Read the model definition and answer for the solid it produces. Units are mm, in the model's axes. Face numbers are marked on the shaded views. A direction names the side the tool comes from. Coordinates: 2 decimals unless noted, no trailing zeros. Write each loop counter-clockwise with the first axis right and the second up, starting at its lowest first coordinate (ties: lowest second). Pieces come first, ordered by that corner, then holes. Notation, with made-up numbers: (20.25, -34) -> (77.25, -34) arc R13 ccw to (77.25, -28) -> close; hole circle Ø4 at (-10.75, 88). An arc over 180 degrees is marked (long way). Answer as a JSON object with one key per item and string values. Group by question number.
(1) Which of the six approach directions +Z, -Z, +X, -X, +Y, -Y give full straight-line access (tool end or side, diameter ignored) to the marked faces 1 and 2?
(2) Find section B-B (x = 23.5). Give the vertices of the cut face in (y, z), then the cut area to 3 significant figures.
(3) Find section C-C (z = 12). Give the vertices of the cut face in (x, y).
(4) For a pull along X with two mould halves and no side action, classify the marked faces 3, 4 and 5 as +X half, -X half, draft (parallel to the pull), parting line (faces both ways), or undercut.
(5) Find section D-D (y = -1.5). Give the vertices of the cut face in (x, z) (3 decimals).
(6) Find section A-A (x = 17.56). Give the vertices of the cut face in (y, z) (3 decimals), then the cut area to 3 significant figures.
(7) Straight lines are drawn through the part: L1, parallel to Z at x = 17.56, y = -1.7 (3 decimals); L2, parallel to Z at x = 26, y = -1.3; L3, parallel to X at y = -2.1, z = 7. For each, find the intervals that lie inside material, in ascending order.
from build123d import *

# Parameters (mm, degrees)
SKETCH_W        = 35.12
SKETCH_H        = 18.62
PAD_DEPTH       = 2.6
SKETCH002_W     = 24.92
SKETCH002_H     = 12.92
POCKET_DEPTH    = 2.6
SKETCH003_R     = 0.5
SKETCH003_W     = 2.01
SKETCH003_H     = 3.5
POCKET001_DEPTH = 5


with BuildPart() as part:
    # Sketch → Pad (new body)
    with BuildSketch(Plane.XZ):
        with Locations((17.56, 9.31)):
            Rectangle(SKETCH_W, SKETCH_H)
    extrude(amount=PAD_DEPTH)

    # Sketch002 (on Face6 of Pad) → Pocket (cut)
    with BuildSketch(Plane.XZ.offset(2.6)):
        with Locations((17.56, 9.31)):
            Rectangle(SKETCH002_W, SKETCH002_H)
    extrude(amount=-POCKET_DEPTH, mode=Mode.SUBTRACT)

    # Sketch003 (on Face4 of Pocket) → Pocket001 (cut)
    with BuildSketch(Plane(origin=(0, 0, 0), x_dir=(1, 0, 0), z_dir=(0, 1, 0))):
        with Locations((17.56, -1.425)):
            Circle(SKETCH003_R)
        with Locations((27.953742, -8.544061)):
            Rectangle(SKETCH003_W, SKETCH003_H)
    extrude(amount=-POCKET001_DEPTH, mode=Mode.SUBTRACT)


solid = part.part
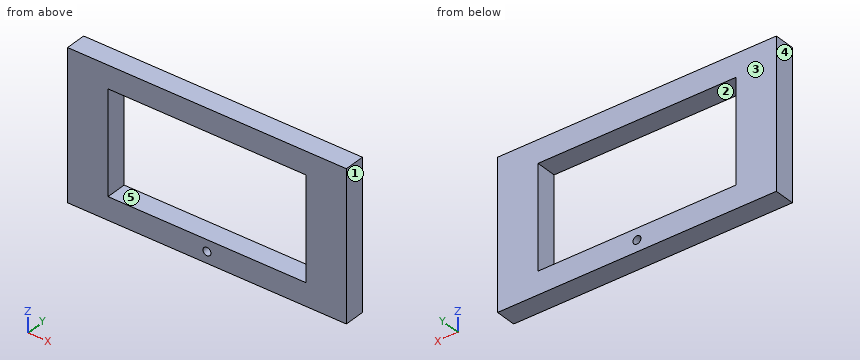
Results below:
{
 "1": {"face 1": "+Z, -Z, +X, +Y, -Y", "face 2": "+Y, -Y"},
 "2": {"outline": "(-2.6, 0) -> (0, 0) -> (0, 2.85) -> (-2.6, 2.85) -> close; (-2.6, 15.77) -> (0, 15.77) -> (0, 18.62) -> (-2.6, 18.62) -> close", "area": "14.8 mm2"},
 "3": {"outline": "(0, -2.6) -> (5.1, -2.6) -> (5.1, 0) -> (0, 0) -> close; (30.02, -2.6) -> (35.12, -2.6) -> (35.12, 0) -> (30.02, 0) -> close"},
 "4": {"face 3": "draft", "face 4": "-X half", "face 5": "undercut"},
 "5": {"outline": "(0, 0) -> (35.12, 0) -> (35.12, 18.62) -> (0, 18.62) -> close; hole (5.1, 2.85) -> (30.02, 2.85) -> (30.02, 15.77) -> (5.1, 15.77) -> close; hole circle Ø1 at (17.56, 1.425)"},
 "6": {"outline": "(-2.6, 0) -> (0, 0) -> (0, 0.925) -> (-2.6, 0.925) -> close; (-2.6, 1.925) -> (0, 1.925) -> (0, 2.85) -> (-2.6, 2.85) -> close; (-2.6, 15.77) -> (0, 15.77) -> (0, 18.62) -> (-2.6, 18.62) -> close", "area": "12.2 mm2"},
 "7": {"L1": "z = 0 to 0.925, 1.925 to 2.85, 15.77 to 18.62", "L2": "z = 0 to 2.85, 15.77 to 18.62", "L3": "x = 0 to 5.1, 30.02 to 35.12"}
}
